```python
from build123d import *

# Parameters (mm, degrees)
SKETCH_1_R      = 2
SKETCH_1_R_2    = 3
EXTRUDE_1_DEPTH = 1
FILLET_1_R      = 2


with BuildPart() as part:
    # Sketch 1 → Extrude 1 (new body)
    with BuildSketch(Plane(origin=(0, 0, 0), x_dir=(1, 0, 0), z_dir=(0, 1, 0))):
        with BuildLine():
            Line((-18.072575848, 120.933670434), (-20, 125))
            Line((-20, 125), (-32.5, 125))
            Line((-32.5, 125), (-32.5, 0))
            Line((-32.5, 0), (32.5, 0))
            Line((32.5, 0), (32.5, 125))
            Line((32.5, 125), (20, 125))
            Line((20, 125), (18.072575848, 120.933670434))
            ThreePointArc((18.072575848, 120.933670434), (0, 109.5), (-18.072575848, 120.933670434))
        make_face()
        with Locations(Location((-18, 7, 0), (0, 0, 270))):
            Circle(SKETCH_1_R, mode=Mode.SUBTRACT)
        with Locations(Location((18, 7, 0), (0, 0, 90))):
            Circle(SKETCH_1_R, mode=Mode.SUBTRACT)
        with Locations(Location((0, 83.51, 0), (0, 0, 270))):
            Circle(SKETCH_1_R_2, mode=Mode.SUBTRACT)
        with BuildLine():
            Line((-4, 35.690566512), (4, 35.690566512))
            ThreePointArc((4, 35.690566512), (5.5, 34.190566512), (4, 32.690566512))
            Line((4, 32.690566512), (-4, 32.690566512))
            ThreePointArc((-4, 32.690566512), (-5.5, 34.190566512), (-4, 35.690566512))
        make_face(mode=Mode.SUBTRACT)
        with BuildLine():
            Line((-4, 45.340566355), (4, 45.340566355))
            ThreePointArc((4, 45.340566355), (5.5, 43.840566355), (4, 42.340566355))
            Line((4, 42.340566355), (-4, 42.340566355))
            ThreePointArc((-4, 42.340566355), (-5.5, 43.840566355), (-4, 45.340566355))
        make_face(mode=Mode.SUBTRACT)
        with BuildLine():
            Line((-4, 54.990566199), (4, 54.990566199))
            ThreePointArc((4, 54.990566199), (5.5, 53.490566199), (4, 51.990566199))
            Line((4, 51.990566199), (-4, 51.990566199))
            ThreePointArc((-4, 51.990566199), (-5.5, 53.490566199), (-4, 54.990566199))
        make_face(mode=Mode.SUBTRACT)
        with BuildLine():
            Line((-4, 64.640566042), (4, 64.640566042))
            ThreePointArc((4, 64.640566042), (5.5, 63.140566042), (4, 61.640566042))
            Line((4, 61.640566042), (-4, 61.640566042))
            ThreePointArc((-4, 61.640566042), (-5.5, 63.140566042), (-4, 64.640566042))
        make_face(mode=Mode.SUBTRACT)
    extrude(amount=EXTRUDE_1_DEPTH)

    # Fillet 1
    fillet_1_edges = [part.edges().sort_by_distance(p)[0] for p in [
        (20, 0.5, -125),
        (32.5, 0.5, -125),
        (32.5, 0.5, 0),
        (-32.5, 0.5, 0),
        (-32.5, 0.5, -125),
        (-20, 0.5, -125),
    ]]
    fillet(fillet_1_edges, radius=FILLET_1_R)


solid = part.part
```
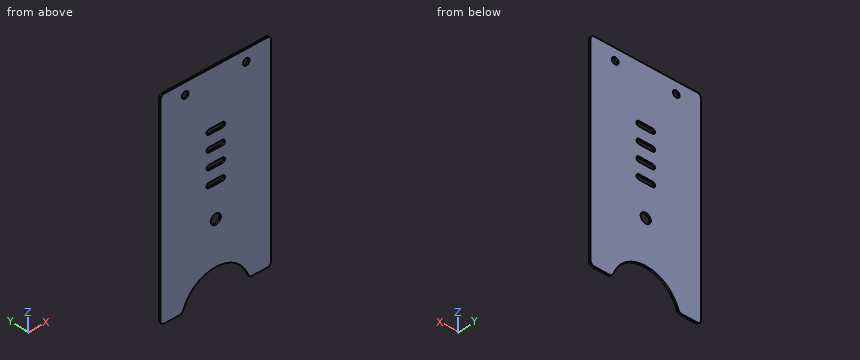
Can you work these out from the model? Positions are in its coordinate system, mm. Give positions to 0.01 mm unless a question says otherwise; leave off trailing zeros. Loops run counter-clockwise (first coordinate to the right, second up) from the corner with the lowest first, then second, coordinate; pieces in that order, holes last. Notation, with made-up numbers: M 40,0 L 54,0 A9 cw 54,8 Z; hole C -27.5,-25.75 d11. An arc over 180 degrees is marked long. Answer in a Markdown table with one row per item.
1. Suppose I cut it at D-D on x = -14. Write out the boundary of the cut face in (y, z).
Taken from the geometry:
| item | result |
|---|---|
| outline | M 0,-115.22 L 1,-115.22 L 1,0 L 0,0 Z |
2. If I drill on line 1 along X through (y, z) = (0.4, -7); line 2 along X through (y, z) = (0.3, -83.51); line 3 along X through (y, z) = (0.5, -117.5), over which ranges is the centre line in solid material (lowest first)?
Taken from the geometry:
| item | result |
|---|---|
| line 1 | x = -32.5 to -20, -16 to 16, 20 to 32.5 |
| line 2 | x = -32.5 to -3, 3 to 32.5 |
| line 3 | x = -32.5 to -16, 16 to 32.5 |
3. Suppose I cut it at A-A on z = -7. Write out the boundary of the cut face in (x, y), plus the area to 3 significant figures.
Taken from the geometry:
| item | result |
|---|---|
| outline | M -32.5,0 L -20,0 L -20,1 L -32.5,1 Z; M -16,0 L 16,0 L 16,1 L -16,1 Z; M 20,0 L 32.5,0 L 32.5,1 L 20,1 Z |
| area | 57.0 mm² |
4. Suppose I cut it at B-B on x = 0. Write out the boundary of the cut face in (y, z).
Taken from the geometry:
| item | result |
|---|---|
| outline | M 0,-109.5 L 1,-109.5 L 1,-86.51 L 0,-86.51 Z; M 0,-80.51 L 1,-80.51 L 1,-64.64 L 0,-64.64 Z; M 0,-61.64 L 1,-61.64 L 1,-54.99 L 0,-54.99 Z; M 0,-51.99 L 1,-51.99 L 1,-45.34 L 0,-45.34 Z; M 0,-42.34 L 1,-42.34 L 1,-35.69 L 0,-35.69 Z; M 0,-32.69 L 1,-32.69 L 1,0 L 0,0 Z |
5. Suppose I cut it at C-C on y = 0.6. Count the separate pieces of the cut face and the enclosed holes in it, plus the area to 3 significant figures.
Taken from the geometry:
| item | result |
|---|---|
| separate pieces | 1 |
| enclosed holes | 7 |
| area | 7,490 mm² |
